```python
from build123d import *

# Parameters (mm, degrees)
SKETCH1_R           = 1.8
SKETCH1_R_2         = 1.6
SKETCH1_R_3         = 2.5
BOSS_EXTRUDE1_DEPTH = 5


with BuildPart() as part:
    # Sketch1 → Boss-Extrude1 (new body)
    with BuildSketch(Plane(origin=(0, 0, 0), x_dir=(1, 0, 0), z_dir=(0, 1, 0))):
        with BuildLine():
            Line((-40.201849804, 94.840698314), (89.589997394, 224.632545513))
            ThreePointArc((89.589997394, 224.632545513), (96.07846437, 228.968000539), (103.732133018, 230.490409889))
            Line((103.732133018, 230.490409889), (196.158539889, 230.490409889))
            ThreePointArc((196.158539889, 230.490409889), (203.812208536, 228.968000539), (210.300675513, 224.632545513))
            Line((210.300675513, 224.632545513), (238.082421443, 196.850799582))
            ThreePointArc((238.082421443, 196.850799582), (242.41787647, 190.362332606), (243.940285819, 182.708663958))
            Line((243.940285819, 182.708663958), (243.940285819, 90.282257087))
            ThreePointArc((243.940285819, 90.282257087), (242.41787647, 82.62858844), (238.082421443, 76.140121463))
            Line((238.082421443, 76.140121463), (108.290574245, -53.651725735))
            ThreePointArc((108.290574245, -53.651725735), (101.802107268, -57.987180761), (94.148438621, -59.509590111))
            Line((94.148438621, -59.509590111), (13.035740249, -59.509590111))
            ThreePointArc((13.035740249, -59.509590111), (5.382071602, -57.987180761), (-1.106395375, -53.651725735))
            Line((-1.106395375, -53.651725735), (-40.201849804, -14.556271305))
            ThreePointArc((-40.201849804, -14.556271305), (-44.537304831, -8.067804329), (-46.059714181, -0.414135682))
            Line((-46.059714181, -0.414135682), (-46.059714181, 80.698562691))
            ThreePointArc((-46.059714181, 80.698562691), (-44.537304831, 88.352231338), (-40.201849804, 94.840698314))
        make_face()
        with Locations((-24.896763277, -15.719222209)):
            Circle(SKETCH1_R, mode=Mode.SUBTRACT)
        with Locations((-2.269346279, -38.346639207)):
            Circle(SKETCH1_R, mode=Mode.SUBTRACT)
        with Locations((204.912940609, 214.090481676)):
            Circle(SKETCH1_R, mode=Mode.SUBTRACT)
        with Locations((227.540357607, 191.463064678)):
            Circle(SKETCH1_R, mode=Mode.SUBTRACT)
        with Locations((-26.310976839, 30.949825349)):
            Circle(SKETCH1_R_2, mode=Mode.SUBTRACT)
        with Locations((44.39970128, -39.76085277)):
            Circle(SKETCH1_R_2, mode=Mode.SUBTRACT)
        with Locations((111.574845492, 27.414291443)):
            Circle(SKETCH1_R_2, mode=Mode.SUBTRACT)
        with Locations((40.864167374, 98.124969562)):
            Circle(SKETCH1_R_2, mode=Mode.SUBTRACT)
        with Locations((-36.197611828, 26.694324714)):
            Circle(SKETCH1_R_2, mode=Mode.SUBTRACT)
        with Locations((41.584134103, -51.087421217)):
            Circle(SKETCH1_R_2, mode=Mode.SUBTRACT)
        with Locations((63.491584372, 96.710755999)):
            Circle(SKETCH1_R_2, mode=Mode.SUBTRACT)
        with Locations((132.788048928, 27.414291443)):
            Circle(SKETCH1_R_2, mode=Mode.SUBTRACT)
        with Locations((177.335776143, 71.962018658)):
            Circle(SKETCH1_R_2, mode=Mode.SUBTRACT)
        with Locations((108.039311586, 141.258483214)):
            Circle(SKETCH1_R_2, mode=Mode.SUBTRACT)
        with Locations((161.966151733, 190.235575893)):
            Circle(SKETCH1_R_2, mode=Mode.SUBTRACT)
        with Locations((203.685451823, 148.516275803)):
            Circle(SKETCH1_R_2, mode=Mode.SUBTRACT)
        with Locations((223.837995087, 168.668819067)):
            Circle(SKETCH1_R_2, mode=Mode.SUBTRACT)
        with Locations((182.118694997, 210.388119157)):
            Circle(SKETCH1_R_2, mode=Mode.SUBTRACT)
        with Locations((89.841260052, 210.741672547)):
            Circle(SKETCH1_R_2, mode=Mode.SUBTRACT)
        with Locations((224.191548478, 76.391384122)):
            Circle(SKETCH1_R_2, mode=Mode.SUBTRACT)
        with Locations((65.246851643, 157.862992891)):
            Circle(SKETCH1_R_2, mode=Mode.SUBTRACT)
        with Locations((87.874268641, 180.490409889)):
            Circle(SKETCH1_R_2, mode=Mode.SUBTRACT)
        with Locations((142.874268641, 221.348274265)):
            Circle(SKETCH1_R_2, mode=Mode.SUBTRACT)
        with Locations((234.798150196, 129.424392711)):
            Circle(SKETCH1_R_2, mode=Mode.SUBTRACT)
        with Locations((28.940285819, 139.941203378)):
            Circle(SKETCH1_R_3, mode=Mode.SUBTRACT)
        with Locations((28.940285819, 124.941203378)):
            Circle(SKETCH1_R_3, mode=Mode.SUBTRACT)
        with BuildLine():
            Line((121.661065206, 193.064003018), (142.874268641, 171.850799582))
            ThreePointArc((142.874268641, 171.850799582), (142.874268641, 157.708663958), (128.732133018, 157.708663958))
            Line((128.732133018, 157.708663958), (107.518929582, 178.921867394))
            ThreePointArc((107.518929582, 178.921867394), (107.518929582, 193.064003018), (121.661065206, 193.064003018))
        make_face(mode=Mode.SUBTRACT)
        with BuildLine():
            Line((185.300675513, 129.424392711), (206.513878948, 108.211189275))
            ThreePointArc((206.513878948, 108.211189275), (206.513878948, 94.069053651), (192.371743324, 94.069053651))
            Line((192.371743324, 94.069053651), (171.158539889, 115.282257087))
            ThreePointArc((171.158539889, 115.282257087), (171.158539889, 129.424392711), (185.300675513, 129.424392711))
        make_face(mode=Mode.SUBTRACT)
        Polygon((63.47908469, 166.701827656), (74.085686408, 156.095225938), (89.642035594, 171.651575124), (79.035433877, 182.258176842), align=None, mode=Mode.SUBTRACT)
    extrude(amount=BOSS_EXTRUDE1_DEPTH)


solid = part.part
```
Geometry check sheet. Reference: the model listing, model coordinates, mm. A direction names the side the tool comes from. Coordinates: 2 decimals unless noted, no trailing zeros. Loops run counter-clockwise (first coordinate to the right, second up) from the corner with the lowest first, then second, coordinate; pieces in that order, holes last.
Item 1: Sectioned sample at C-C, the plane y = 3.3. Count the separate pieces of the cut face and the enclosed holes in it, then the cut area to 3 significant figures.
Item 2: Sectioned sample at B-B, the plane z = 7. Record the boundary of the cut face in (x, y), then the cut area to 3 significant figures.
Item 3: Access from +Z, -Z, +X, -X, +Y, -Y to the whole of each face (thin tool, end or side, straight path). Record for faces 4 (the face through (118.27, 2.46, -168.17)), 5 (the face through (23.79, 2.46, -158.83)).
Item 4: Thickness scan on line 1 (Z direction, x = 87.5, y = 4.3); line 2 (Z direction, x = 206.5, y = 2.8); line 3 (Z direction, x = 71, y = 2.7). Record the ranges inside material, lowest first.
Item 5: Release check for a two-part mould opening along Z. For faces 1 (the face through (68.71, 2.46, -161.47)), 2 (the face through (101, 0, -88)), 3 (the face through (-20.38, 2.46, 34.38)) record: released by +Z, released by -Z, zero draft, split by the parting line, or undercut.
Item 6: Sectioned sample at A-A, the plane x = 116.5. Record the boundary of the cut face in (y, z), then the cut area to 3 significant figures.
Item 7: Sectioned sample at D-D, the plane x = -16. Record the boundary of the cut face in (y, z), then the cut area to 3 significant figures.
Item 8: Go/stop test with flat-tipped pins: pin 1 Ø6 at (x, z) = (175, -181) entering from -Y; pin 2 Ø2 at (y, z) = (0.5, 1) entering from +X; pin 3 Ø1 at (x, y) = (208.5, 1.5) entering from -Z. Record where each tip stops, or that it passes through.
Check result:
1. separate pieces: 1
1. enclosed holes: 29
1. area: 59,500 mm2
2. outline: (-44.94, 0) - (154.94, 0) - (154.94, 5) - (-44.94, 5) - close
2. area: 999 mm2
3. face 4: +Y, -Y
3. face 5: -Z, -X, +Y, -Y
4. line 1: z = -222.54 to -182.05, -178.93 to -173.79, -169.51 to 59.51
4. line 2: z = -227.61 to -214.94, -213.24 to -108.23, -94.06 to -44.56
4. line 3: z = -206.04 to -174.22, -159.18 to 59.51
5. face 1: undercut
5. face 2: zero draft
5. face 3: released by +Z
6. outline: (0, -230.49) - (5, -230.49) - (5, -195.81) - (0, -195.81) - close; (0, -169.94) - (5, -169.94) - (5, 45.44) - (0, 45.44) - close
6. area: 1,250 mm2
7. outline: (0, -119.04) - (5, -119.04) - (5, 38.76) - (0, 38.76) - close
7. area: 789 mm2
8. pin 1: stops at y = 0
8. pin 2: stops at x = 161.94
8. pin 3: stops at z = -226.61
